Build history of the part. All positions in model axes, mm. A direction names the side the tool comes from. Give positions to 0.01 mm unless a question says otherwise; leave off trailing zeros. Loops run counter-clockwise (first coordinate to the right, second up) from the corner with the lowest first, then second, coordinate; pieces in that order, holes last.
1) Flat gauge pins, fed straight in: P1, Ø15, axis at x = -31.5, y = 45, coming from the -Z side; P2, Ø8, axis at x = -55.5, z = -97, coming from the +Y side; P3, Ø2, axis at x = -74, y = 22.5, coming from the +Z side. Where does each tip first touch, or does it go through?
2) Two-plate mould, pull along Z, no slides. Class faces 1 (the cylindrical face through (64.862, 21.197, -36.056)), 2 (the flat face through (-1, 45, 0)), 3 (the flat face through (0, 0, 40)): +Z half, -Z half, draft (parallel to the pull), parting line (faces both ways), or undercut.
3) Band-saw the part on D-D on x = 41. List the corners of the cut face in (y, z).
4) Band-saw the part on A-A on x = -50. List the corners of the cut face in (y, z).
5) Band-saw the part on C-C on y = 0. List the corners of the cut face in (x, z), then the cut area to 3 significant figures.
6) 3-axis set-ups, long thin cutter, end or side, ignore diameter. For faces 4 (the flat face through (-1, -32, 30)), 5 (the flat face through (-60, 17.5, -33)), 6 (the cylindrical face through (52.41, 0.25, -5.26)), 7 (the flat face through (1, 25, -74)), 8 (the flat face through (75, 0, -104)): which of +Z, -Z, +X, -X, +Y, -Y reach the whole face in a straight line?
7) Wall check: line 1 (X direction, y = -19.75, z = -25); line 2 (Z direction, x = -50, y = -2); line 3 (Y direction, x = 55.5, z = -41). Give the ranges that are in metal, low to high.
8) Band-saw the part on B-B on z = -25. List the corners of the cut face in (x, y).
Autodesk Inventor part; units mm, degrees
ref_plane "YZ Plane" through (0, 0, 0) normal (1, 0, 0) x (0, 1, 0)
ref_plane "XZ Plane" through (0, 0, 0) normal (0, 1, 0) x (-1, 0, 0)
ref_plane "XY Plane" through (0, 0, 0) normal (0, 0, 1) x (1, 0, 0)
sketch "草图1" plane through (0, 0, 0) normal (0, 0, 1) x (1, 0, 0)
  circle A0 centre (0, 0) radius 75
  dimension "d0" = 150
extrude "拉伸1" add sketch "草图1" along normal blind 30
sketch "草图2" plane through (0, 0, 30) normal (0, 0, 1) x (1, 0, 0)
  circle A0 centre (0, 0) radius 30
  dimension "d3" = 60
extrude "拉伸2" add sketch "草图2" along normal blind 10
sketch "草图3" plane through (0, 0, 0) normal (0, 0, -1) x (-1, 0, 0)
  circle A0 centre (0, 0) radius 75
  line L0 (-75, 25) -> (75, 25)
  line L1 (75, 25) -> (75, -25)
  line L2 (75, -25) -> (-75, -25)
  line L3 (-75, -25) -> (-75, 25)
  line L4 (-75, 25) -> (75, -25) construction
  line L5 (75, 25) -> (-75, -25) construction
  dimension "d21" = 50
  dimension "d22" = 150
extrude "拉伸3" add sketch "草图3" along normal blind 150 contours A0 L2 L0 | L1 L2 A0 | A0 L0 L1 | A0 L3 L0 | L2 L3 A0
sketch "草图4" plane through (-70, 25, 0) normal (0, 1, 0) x (1, 0, 0)
  circle A0 centre (120, 125) radius 15
  circle A1 centre (20, 125) radius 15
  line L0 (145, 0) -> (145, 150)
  arc A2 (145, 125) -> (95, 125) centre (120, 125) ccw
  line L1 (-5, 150) -> (145, 150)
  arc A3 (45, 125) -> (-5, 125) centre (20, 125) ccw
  line L2 (145, 125) -> (145, 150)
  line L3 (120, 150) -> (20, 150)
  line L4 (-5, 0) -> (-5, 150)
  line L5 (-5, 150) -> (20, 150)
  line L6 (-5, 150) -> (-5, 125)
  line L7 (95, 125) -> (45, 125)
  point P0 (70, 0)
  dimension "d12" = 30
  dimension "d13" = 30
  dimension "d23" = 100
  dimension "d24" = 25
extrude "拉伸4" cut sketch "草图4" against normal through all
sketch "草图5" plane through (-70.7107, -25, 0) normal (0, -1, 0) x (1, 0, 0)
  line L0 (-4.2893, 0) -> (-4.2893, -125)
  line L1 (145.7107, 0) -> (145.7107, -125)
  line L2 (0, 0) -> (141.4214, 0)
  circle A0 centre (-4.2893, -25) radius 25
  circle A1 centre (145.7107, -25) radius 25
  circle A2 centre (-4.2893, -25) radius 15
  circle A3 centre (145.7107, -25) radius 15
  point P0 (70.7107, 0)
  dimension "d34" = 30
  dimension "d35" = 30
extrude "拉伸5" add sketch "草图5" against normal up to surface (50 mm away) contours A0 L0 A2 | L0 A2 A0 | A1 L1 A3 | L1 A3 A1
extrude "拉伸6" cut sketch "草图5" against normal through all contours A2 L0 | L0 A2 | A3 L1 | L1 A3
sketch "草图6" plane through (0, 0, 0) normal (0, 1, 0) x (-1, 0, 0)
  circle A0 centre (75, -25) radius 15
  circle A1 centre (75, -25) radius 30
  circle A2 centre (-75, -25) radius 15
  circle A3 centre (-75, -25) radius 30
  point P0 (0, 0)
  dimension "d40" = 60
  dimension "d41" = 60
extrude "拉伸7" cut sketch "草图6" along normal mid plane 35
chamfer "倒角1" distance 40 angle 45 2 edges at (-75, 0, -55) (75, 0, -55)
equation "\"d36\" = d13"
equation "\"d38\" = d13"
properties part number "Pam" material "钢，高强度，低合金"
Findings below:
1. P1: stops at z = 0
1. P2: stops at y = 25
1. P3: stops at z = 0
2. face 1: undercut
2. face 2: -Z half
2. face 3: +Z half
3. outline: (-62.8, 0) - (-25, 0) - (-25, -113) - (25, -113) - (25, 0) - (62.8, 0) - (62.8, 30) - (-62.8, 30) - close; (-25, -148.32) - (25, -148.32) - (25, -137) - (-25, -137) - close
4. outline: (-55.9, 0) - (-25, 0) - (-25, -110) - (25, -110) - (25, 0) - (55.9, 0) - (55.9, 30) - (-55.9, 30) - close; (-25, -150) - (25, -150) - (25, -140) - (-25, -140) - close; hole (-17.5, -39.1) - (17.5, -39.1) - (17.5, -8.42) - (-17.5, -8.42) - close
5. outline: (-75, -125) arc R25 ccw to (-25, -125) - (25, -125) arc R25 ccw to (75, -125) - (75, -95) - (45.19, -28.33) arc R30 cw to (75, 5) - (75, 30) - (30, 30) - (30, 40) - (-30, 40) - (-30, 30) - (-75, 30) - (-75, 5) arc R30 cw to (-45.19, -28.33) - (-75, -95) - close; hole circle Ø30 at (-50, -125); hole circle Ø30 at (50, -125)
5. area: 20,800 mm2
6. face 4: +Z
6. face 5: -X
6. face 6: +X
6. face 7: -Z, +X, -X, +Y
6. face 8: -Z, +X, +Y, -Y
7. line 1: x = -100 to -90, -60 to 60, 90 to 100
7. line 2: z = -150 to -140, -110 to -39.1, -8.42 to 30
7. line 3: y = -25 to -17.5, 17.5 to 25
8. outline: (-100, -25) - (-90, -25) - (-90, -17.5) - (-100, -17.5) - close; (-100, 17.5) - (-90, 17.5) - (-90, 25) - (-100, 25) - close; (-60, -25) - (60, -25) - (60, -17.5) - (45, -17.5) - (45, 17.5) - (60, 17.5) - (60, 25) - (-60, 25) - (-60, 17.5) - (-45, 17.5) - (-45, -17.5) - (-60, -17.5) - close; (90, -25) - (100, -25) - (100, -17.5) - (90, -17.5) - close; (90, 17.5) - (100, 17.5) - (100, 25) - (90, 25) - close
